Geometry: final body of the model. Coordinates: model frame, mm. Round coordinates to 2 decimals unless told otherwise and drop trailing zeros. Write each loop counter-clockwise with the first axis right and the second up, starting at its lowest first coordinate (ties: lowest second). Pieces come first, ordered by that corner, then holes. Notation, with made-up numbers: M -6,-0.5 L 1,-0.5 A7 ccw 1,3.5 Z; hole C 3.25,-24 d2. An arc over 180 degrees is marked long. Use one line per item in the form item = value. Start each with the question number.
Item 1: Section query A-A (z = 1.05). State how many separate pieces and enclosed holes the cut face has, and give its area (3 significant figures).
Item 2: Pin query (flat end, axial travel): pin 1 Ø1.6 at (x, y) = (81.06, 34) entering from -Z; pin 2 Ø0.8 at (x, z) = (64, 0.5) entering from +Y; pin 3 Ø0.8 at (y, z) = (91.5, 1) entering from -X. Return the tip coordinate at first contact, or that it passes through.
Item 3: Ray query, probe 1 along X at (y, z) = (134, 0.4); probe 2 along X at (y, z) = (-56, 1); probe 3 along Y at (x, z) = (132, 0.3). Return the intervals inside material, ascending.
Item 4: Section query B-B (y = 71). Return loops of the section in (x, z), and give its area (3 significant figures).
Item 5: Section query C-C (x = 48). Return loops of the section in (y, z).
Autodesk Inventor part; units mm, degrees
ref_plane "РабПлоскость1" through (0, 0, 0) normal (0, 0, 1) x (1, 0, 0)
ref_plane "РабПлоскость2" through (0, 0, 0) normal (0, 0, 1) x (1, 0, 0)
ref_plane "YZ Plane" through (0, 0, 0) normal (1, 0, 0) x (0, 1, 0)
ref_plane "РабПлоскость1" through (0, 0, 0) normal (0, 0, 1) x (1, 0, 0)
ref_plane "РабПлоскость2" through (0, 0, 0) normal (0, 0, 1) x (1, 0, 0)
sketch "Эскиз2" plane through (0, 0, 0) normal (0, 0, 1) x (1, 0, 0)
  line L0 (164.5082, 55.3787) -> (164.5082, 22.6213)
  line L1 (152.0082, 55.3787) -> (164.5082, 55.3787)
  spline S0 degree 4 poles (142.0082, 66.7804) (141.9936, 65.5806) (142.2897, 63.8407) (143.0904, 61.8123) (144.7867, 59.6039) (146.7684, 57.7973) (148.9036, 56.5519) (150.6395, 55.9298) (152.0082, 55.3787) knots 0 0 0 0 0 0.305903 0.428365 0.551581 0.676311 1 1 1 1 1
  line L2 (142.0082, 89.6988) -> (142.0082, 66.7804)
  spline S1 degree 4 poles (142.0976, 90.5077) (142.1863, 90.3272) (142.1406, 90.1079) (142.065, 89.9075) (142.0082, 89.6988) knots 0 0 0 0 0 1 1 1 1 1
  ellipse E0 centre (144.0082, 89.6716) end of major axis (144.0082, 92.5) minor radius 2 (144.0082, 92.5) -> (142.0976, 90.5077) ccw
  line L3 (144.0082, 92.5) -> (149.4338, 92.5)
  line L4 (149.4338, 92.5) -> (149.4338, 92.525)
  line L5 (149.4338, 92.525) -> (142.946, 92.525)
  ellipse E1 centre (142.946, 98.525) end of major axis (136.7344, 98.525) minor radius 6 (136.7344, 98.525) -> (142.946, 92.525) ccw
  line L6 (136.7344, 98.525) -> (136.7344, 100.025)
  ellipse E2 centre (142.946, 100.025) end of major axis (136.7344, 100.025) minor radius 6 (142.946, 106.025) -> (136.7344, 100.025) ccw
  line L7 (142.946, 106.025) -> (149.4338, 106.025)
  line L8 (149.4338, 106.025) -> (149.4338, 106.05)
  line L9 (149.4338, 106.05) -> (144.0082, 106.05)
  ellipse E3 centre (144.0082, 108.8784) end of major axis (144.0082, 106.05) minor radius 2 (142.0976, 108.0423) -> (144.0082, 106.05) ccw
  spline S2 degree 4 poles (142.0082, 108.8512) (142.0222, 108.6489) (142.0418, 108.4466) (142.067, 108.2444) (142.0976, 108.0423) knots 0 0 0 0 0 1 1 1 1 1
  line L10 (142.0082, 108.8512) -> (142.0082, 139)
  arc A0 (142.0082, 139) -> (137.0082, 144) centre (137.0082, 139) ccw
  line L11 (137.0082, 144) -> (27.0082, 144)
  arc A1 (27.0082, 144) -> (22.0082, 139) centre (27.0082, 139) ccw
  line L12 (22.0082, 139) -> (22.0082, 108.8512)
  spline S3 degree 4 poles (21.9188, 108.0423) (21.9596, 108.2417) (21.9876, 108.4433) (22.0035, 108.6467) (22.0082, 108.8512) knots 0 0 0 0 0 1 1 1 1 1
  ellipse E4 centre (20.0082, 108.8784) end of major axis (20.0082, 106.05) minor radius 2 (20.0082, 106.05) -> (21.9188, 108.0423) ccw
  line L13 (14.5826, 106.05) -> (20.0082, 106.05)
  line L14 (14.5826, 106.025) -> (14.5826, 106.05)
  line L15 (21.0704, 106.025) -> (14.5826, 106.025)
  ellipse E5 centre (21.0704, 100.025) end of major axis (27.282, 100.025) minor radius 6 (27.282, 100.025) -> (21.0704, 106.025) ccw
  ellipse E6 centre (21.0704, 98.525) end of major axis (27.282, 98.525) minor radius 6 (21.0704, 92.525) -> (27.282, 98.525) ccw
  line L16 (14.5826, 92.525) -> (21.0704, 92.525)
  line L17 (14.5826, 92.5) -> (14.5826, 92.525)
  line L18 (20.0082, 92.5) -> (14.5826, 92.5)
  ellipse E7 centre (20.0082, 89.6716) end of major axis (20.0082, 92.5) minor radius 2 (21.9188, 90.5077) -> (20.0082, 92.5) ccw
  spline S4 degree 4 poles (22.0082, 89.6988) (22.0001, 89.9001) (21.9823, 90.1037) (21.9553, 90.3071) (21.9188, 90.5077) knots 0 0 0 0 0 1 1 1 1 1
  line L19 (22.0082, 89.6988) -> (22.0082, 66.7804)
  spline S5 degree 4 poles (12.0082, 55.3787) (13.3543, 55.9133) (15.0972, 56.5843) (17.1914, 57.7632) (19.2093, 59.6353) (20.8508, 61.7502) (21.742, 63.9004) (21.9889, 65.5297) (22.0082, 66.7804) knots 0 0 0 0 0 0.323057 0.447569 0.570948 0.693515 1 1 1 1 1
  line L20 (-0.4918, 55.3787) -> (12.0082, 55.3787)
  line L21 (-0.4918, 22.6213) -> (-0.4918, 55.3787)
  line L22 (12.0082, 22.6213) -> (-0.4918, 22.6213)
  spline S6 degree 4 poles (22.0082, 11.2196) (21.9907, 12.4712) (21.7455, 14.1022) (20.8556, 16.2534) (19.2129, 18.3699) (17.1941, 20.2411) (15.0987, 21.4185) (13.3552, 22.0877) (12.0082, 22.6213) knots 0 0 0 0 0 0.306528 0.4291 0.552475 0.676977 1 1 1 1 1
  line L23 (22.0082, -11.6988) -> (22.0082, 11.2196)
  spline S7 degree 4 poles (22.2969, -12.5077) (22.2375, -12.3039) (22.1691, -12.101) (22.0924, -11.8993) (22.0082, -11.6988) knots 0 0 0 0 0 1 1 1 1 1
  ellipse E8 centre (20.3863, -11.6716) end of major axis (20.3863, -14.5) minor radius 2 (20.3863, -14.5) -> (22.2969, -12.5077) ccw
  line L24 (20.3863, -14.5) -> (14.9607, -14.5)
  line L25 (14.9607, -14.5) -> (14.9607, -14.525)
  line L26 (14.9607, -14.525) -> (21.4484, -14.525)
  ellipse E9 centre (21.4484, -20.525) end of major axis (27.6601, -20.525) minor radius 6 (27.6601, -20.525) -> (21.4484, -14.525) ccw
  line L27 (27.6601, -20.525) -> (27.6601, -22.025)
  ellipse E10 centre (21.4484, -22.025) end of major axis (27.6601, -22.025) minor radius 6 (21.4484, -28.025) -> (27.6601, -22.025) ccw
  line L28 (21.4484, -28.025) -> (14.9607, -28.025)
  line L29 (14.9607, -28.025) -> (14.9607, -28.05)
  line L30 (14.9607, -28.05) -> (20.3863, -28.05)
  ellipse E11 centre (20.3863, -30.8784) end of major axis (20.3863, -28.05) minor radius 2 (22.2969, -30.0423) -> (20.3863, -28.05) ccw
  spline S8 degree 4 poles (22.0082, -30.8512) (22.0994, -30.6437) (22.1874, -30.4372) (22.2667, -30.2332) (22.2969, -30.0423) knots 0 0 0 0 0 1 1 1 1 1
  line L31 (22.0082, -30.8512) -> (22.0082, -61)
  arc A2 (22.0082, -61) -> (27.0082, -66) centre (27.0082, -61) ccw
  line L32 (27.0082, -66) -> (137.0082, -66)
  arc A3 (137.0082, -66) -> (142.0082, -61) centre (137.0082, -61) ccw
  line L33 (142.0082, -61) -> (142.0082, -30.8512)
  spline S9 degree 4 poles (142.0976, -30.0423) (142.0618, -30.2424) (142.0345, -30.444) (142.0164, -30.6471) (142.0082, -30.8512) knots 0 0 0 0 0 1 1 1 1 1
  ellipse E12 centre (144.0082, -30.8784) end of major axis (144.0082, -28.05) minor radius 2 (144.0082, -28.05) -> (142.0976, -30.0423) ccw
  line L34 (149.4338, -28.05) -> (144.0082, -28.05)
  line L35 (149.4338, -28.025) -> (149.4338, -28.05)
  line L36 (142.946, -28.025) -> (149.4338, -28.025)
  ellipse E13 centre (142.946, -22.025) end of major axis (136.7344, -22.025) minor radius 6 (136.7344, -22.025) -> (142.946, -28.025) ccw
  line L37 (136.7344, -20.525) -> (136.7344, -22.025)
  ellipse E14 centre (142.946, -20.525) end of major axis (136.7344, -20.525) minor radius 6 (142.0082, -14.5938) -> (136.7344, -20.525) ccw
  spline S10 degree 4 poles (143.3575, -14.5382) (143.017, -14.5392) (142.6788, -14.5494) (142.3414, -14.5663) (142.0082, -14.5938) knots 0 0 0 0 0 1 1 1 1 1
  spline S11 degree 4 poles (143.3575, -14.5382) (143.1143, -14.3292) (142.8382, -14.0321) (142.6629, -13.7922) (142.4735, -13.4852) knots 0 0 0 0 0 1 1 1 1 1
  ellipse E15 centre (144.0082, -11.6716) end of major axis (144.0082, -8.8431) minor radius 2 (142.0976, -12.5077) -> (142.4735, -13.4852) ccw
  spline S12 degree 4 poles (142.0976, -12.5077) (142.0566, -12.3073) (142.0277, -12.1043) (142.0113, -11.9008) (142.0082, -11.6988) knots 0 0 0 0 0 1 1 1 1 1
  line L38 (142.0082, 11.2196) -> (142.0082, -11.6988)
  spline S13 degree 4 poles (152.0082, 22.6213) (150.6678, 22.0949) (148.9359, 21.4381) (146.8415, 20.2599) (144.8098, 18.3825) (143.1469, 16.2574) (142.2323, 14.098) (142.0013, 12.4654) (142.0082, 11.2196) knots 0 0 0 0 0 0.322163 0.446837 0.570623 0.693583 1 1 1 1 1
  line L39 (164.5082, 22.6213) -> (152.0082, 22.6213)
  line L40 (27.282, 98.525) -> (27.282, 100.025)
  line L41 (27.6601, -66) -> (136.7344, -66)
  line L42 (136.7344, -66) -> (136.7344, 55.12)
  line L43 (85.3082, 55.12) -> (27.6601, 55.12)
  line L44 (27.6601, 55.12) -> (27.6601, -66)
  line L45 (49.6082, 55.12) -> (60.6082, 55.12)
  line L46 (85.3082, 55.12) -> (85.3082, 144)
  line L47 (85.3082, 144) -> (136.7344, 144)
  line L48 (136.7344, 144) -> (136.7344, 55.12)
  line L49 (85.3082, 113.52) -> (85.3082, 107.52)
  line L50 (84.3244, 70.87) -> (84.3244, 64.87)
  line L51 (27.6601, 50.12) -> (90.3082, 50.12)
  line L52 (136.7344, 57.0858) -> (136.7344, -61)
  line L53 (136.7344, -61) -> (27.6601, -61)
  line L54 (27.6601, -61) -> (27.6601, 50.12)
  line L55 (90.3082, 50.12) -> (90.3082, 139)
  line L56 (90.3082, 139) -> (136.7344, 139)
  line L57 (136.7344, 139) -> (136.7344, 57.0858)
  point P0 (0, 0)
  point P1 (142.0243, 108.6495)
  point P2 (142.0445, 108.4475)
  point P3 (142.069, 108.2451)
  point P4 (21.9548, 108.2422)
  point P5 (21.9815, 108.4436)
  point P6 (21.9992, 108.6466)
  point P7 (21.9966, 89.8995)
  point P8 (21.9778, 90.1023)
  point P9 (21.9518, 90.3056)
  point P10 (14.1516, 56.2573)
  point P11 (16.0588, 57.2184)
  point P12 (17.7454, 58.3637)
  point P13 (19.1678, 59.6884)
  point P14 (20.3459, 61.2222)
  point P15 (21.2579, 62.9881)
  point P16 (21.8122, 64.8416)
  point P17 (21.8145, 13.1602)
  point P18 (21.2616, 15.0151)
  point P19 (20.35, 16.7819)
  point P20 (19.1713, 18.3166)
  point P21 (17.7482, 19.6409)
  point P22 (16.0609, 20.785)
  point P23 (14.1529, 21.7445)
  point P24 (22.2348, -12.3061)
  point P25 (22.1658, -12.104)
  point P26 (22.0903, -11.9016)
  point P27 (22.102, -30.634)
  point P28 (22.1869, -30.423)
  point P29 (22.2547, -30.224)
  point P30 (142.0651, -30.2427)
  point P31 (142.0392, -30.4442)
  point P32 (142.0201, -30.6471)
  point P33 (143.0157, -14.5425)
  point P34 (142.6767, -14.5533)
  point P35 (142.3406, -14.5702)
  point P36 (143.1122, -14.3072)
  point P37 (142.8714, -14.0419)
  point P38 (142.6642, -13.7743)
  point P39 (142.061, -12.3056)
  point P40 (142.0338, -12.1027)
  point P41 (142.0162, -11.9001)
  point P42 (149.8807, 21.759)
  point P43 (147.9821, 20.8085)
  point P44 (146.2898, 19.6634)
  point P45 (144.8524, 18.3311)
  point P46 (143.6547, 16.7844)
  point P47 (142.7262, 15.0053)
  point P48 (142.1752, 13.1484)
  point P49 (142.1418, 90.326)
  point P50 (142.1248, 90.1256)
  point P51 (142.0712, 89.914)
  point P52 (142.1871, 64.8545)
  point P53 (142.7332, 62.9853)
  point P54 (143.6182, 61.2481)
  point P55 (144.8211, 59.6733)
  point P56 (146.2281, 58.3691)
  point P57 (147.919, 57.2204)
  point P58 (149.8389, 56.2585)
  point P59 (82.0082, 39)
  point P60 (136.7344, -21.275)
  point P61 (27.6601, -21.275)
  dimension "d5" = 0
  dimension "d6" = 0
  dimension "d7" = 0
  dimension "d8" = 0
  dimension "d9" = 0
  dimension "d10" = 5
  dimension "d11" = 5
  dimension "d12" = 0
  dimension "d13" = 5
  dimension "d14" = 0
  dimension "d15" = 5
extrude "Выдавливание1" add sketch "Эскиз2" along normal blind 1.5 contours L37 L42 L53 L44 L27 L51 L55 L56 L48 L6
fillet "Сопряжение1" radius 3 6 edges at (27.6601, 50.12, 0.75) (90.3082, 50.12, 0.75) (90.3082, 139, 0.75) (136.7344, 139, 0.75) (136.7344, -61, 0.75) (27.6601, -61, 0.75)
sketch "Эскиз3" plane through (0, 0, 1.5) normal (0, 0, 1) x (1, 0, 0)
  arc A0 (27.6601, -58) -> (30.6601, -61) centre (30.6601, -58) ccw
  line L0 (30.6601, -61) -> (133.7344, -61)
  arc A1 (133.7344, -61) -> (136.7344, -58) centre (133.7344, -58) ccw
  line L1 (136.7344, -58) -> (136.7344, 136)
  arc A2 (136.7344, 136) -> (133.7344, 139) centre (133.7344, 136) ccw
  line L2 (133.7344, 139) -> (93.3082, 139)
  arc A3 (93.3082, 139) -> (90.3082, 136) centre (93.3082, 136) ccw
  line L3 (90.3082, 136) -> (90.3082, 53.12)
  arc A4 (87.3082, 50.12) -> (90.3082, 53.12) centre (87.3082, 53.12) ccw
  line L4 (87.3082, 50.12) -> (30.6601, 50.12)
  arc A5 (30.6601, 50.12) -> (27.6601, 47.12) centre (30.6601, 47.12) ccw
  line L5 (27.6601, 47.12) -> (27.6601, -58)
  circle A6 centre (32.6601, -56) radius 1.5
  circle A7 centre (32.6601, 45.12) radius 1.5
  circle A8 centre (131.7344, -56) radius 1.5
  circle A9 centre (131.7344, 134) radius 1.5
  circle A10 centre (95.3082, 134) radius 1.5
  point P0 (0, 0)
  dimension "d19" = 5
  dimension "d20" = 3
  dimension "d21" = 5
  dimension "d22" = 3
  dimension "d23" = 3
  dimension "d24" = 3
  dimension "d25" = 3
  dimension "d26" = 5
  dimension "d27" = 5
  dimension "d28" = 5
  dimension "d29" = 5
  dimension "d30" = 5
  dimension "d31" = 5
  dimension "d32" = 5
  dimension "d33" = 5
hole "Отверстие1" at (32.6601, 45.12, 1.5) at (32.6601, -56, 1.5) at (131.7344, -56, 1.5) at (131.7344, 134, 1.5) at (95.3082, 134, 1.5) direction (0, 0, -1) diameter 2.9 end through all
sketch "Эскиз4" plane through (0, 0, 1.5) normal (0, 0, 1) x (1, 0, 0)
  circle A0 centre (73.4444, 34) radius 0.6
  circle A1 centre (75.9844, 34) radius 0.6
  circle A2 centre (78.5244, 34) radius 0.6
  circle A3 centre (81.0644, 34) radius 0.6
  circle A4 centre (83.6044, 34) radius 0.6
  circle A5 centre (86.1444, 34) radius 0.6
  circle A6 centre (88.6844, 34) radius 0.6
  circle A7 centre (91.2244, 34) radius 0.6
  point P0 (0, 0)
extrude "Выдавливание2" cut sketch "Эскиз4" against normal blind 10
properties part number "Motherboard"
Working result:
q1.separate_pieces = 1
q1.enclosed_holes = 13
q1.area = 16,200 mm²
q2.pin_1 = 0
q2.pin_2 = 50.12
q2.pin_3 = 90.31
q3.probe_1 = 90.31 to 93.86, 96.76 to 130.28, 133.18 to 136.73
q3.probe_2 = 27.66 to 31.21, 34.11 to 130.28, 133.18 to 136.73
q3.probe_3 = -61 to -57.43, -54.57 to 132.57, 135.43 to 139
q4.outline = M 90.31,0 L 136.73,0 L 136.73,1.5 L 90.31,1.5 Z
q4.area = 69.6 mm²
q5.outline = M -61,0 L 50.12,0 L 50.12,1.5 L -61,1.5 Z
